Here's how the part is built. I have some questions about the finished solid (model axes, mm). A direction names the side the tool comes from. Coordinates: 2 decimals unless noted, no trailing zeros. Write each loop counter-clockwise with the first axis right and the second up, starting at its lowest first coordinate (ties: lowest second). Pieces come first, ordered by that corner, then holes. Notation, with made-up numbers: (44.25, 54) -> (103.25, 54) arc R25 ccw to (103.25, 70) -> close; hole circle Ø9 at (12.5, 56.5). An arc over 180 degrees is marked (long way). Use a Markdown table: item, result. Add a question column.
Item 1: Imagine slicing it at D-D, the plane z = 12. Write out the boundary of the cut face in (x, y), and give its area (3 significant figures).
Item 2: Imagine slicing it at C-C, the plane z = -13. Write out the boundary of the cut face in (x, y).
Item 3: If I drill on line 1 along X through (y, z) = (4.25, 1); line 2 along Y through (x, z) = (9, 8); line 3 along X through (y, z) = (7.5, -1.5), over which ranges is the centre line in solid material (lowest first)? Write a range as from..to.
Item 4: Imagine slicing it at A-A, the plane x = 0. Write out the boundary of the cut face in (y, z).
Item 5: Will these pins go through, and if not, where does the flat tip stop? pin 1 Ø2.5 at (y, z) = (7.5, 0.5) entering from -X; pin 2 Ø5 at (x, z) = (-12, 6.5) entering from +Y; pin 3 Ø6 at (y, z) = (7, -3) entering from +X.
Item 6: If we mould it in two halves opening along Z, with no side actions, what happens to faces 1 (the cylindrical face through (21.75, 6.45, -4.94)), 2 (the cylindrical face through (-20.66, 6.45, -1.75)), 3 (the flat face through (-30, 1, -9))? For each: pulls with the +Z half, pulls with the -Z half, needs draft (parallel to the pull), parting line crosses it, or undercut.
Item 7: Imagine slicing it at B-B, the plane y = 7.5. Write out the boundary of the cut face in (x, z), and give its area (3 significant figures).
Item 8: On a 3-axis mill with a long thin cutter (end or side, diameter ignored), from which of +Z, -Z, +X, -X, +Y, -Y can I reach the whole of each face in a straight line? I mean faces 4 (the flat face through (-27.7, 6, -5)), 5 (the flat face through (25.7, 6, -3)), 6 (the flat face through (27.7, 6, -5)), 7 (the cylindrical face through (0.609, 6.451, 27.693)), 8 (the flat face through (-15.214, 7, 0)). Say none if no direction works.
Autodesk Inventor part; units mm, degrees
ref_plane "YZ Plane" through (0, 0, 0) normal (1, 0, 0) x (0, 1, 0)
ref_plane "XZ Plane" through (0, 0, 0) normal (0, 1, 0) x (-1, 0, 0)
ref_plane "XY Plane" through (0, 0, 0) normal (0, 0, 1) x (1, 0, 0)
sketch "Sketch1" plane through (0, 0, 0) normal (0, 1, 0) x (-1, 0, 0)
  arc A0 (30, 0) -> (-30, 0) centre (0, 0) ccw
  line L0 (30, 0) -> (30, -18)
  line L1 (-30, 0) -> (-30, -18)
  arc A1 (30, -18) -> (-30, -18) centre (0, -34) ccw
  dimension "d0" = 60
  dimension "d1" = 34
  dimension "d4" = 18
extrude "Extrusion1" add sketch "Sketch1" along normal blind 3
sketch "Sketch2" plane through (0, 3, 0) normal (0, 1, 0) x (1, 0, 0)
  arc A0 (-30, 0) -> (30, 0) centre (0, 0) ccw
  arc A1 (-30, 18) -> (30, 18) centre (0, 34) ccw
  line L0 (-30, 18) -> (-30, 0)
  line L1 (30, 0) -> (30, 18)
  arc A2 (-27.7, 0) -> (27.7, 0) centre (0, 0) ccw
  line L2 (-27.7, 0) -> (-27.7, 10.5394)
  arc A3 (-27.7, 10.5394) -> (27.7, 10.5394) centre (0, 34) ccw
  line L3 (27.7, 10.5394) -> (27.7, 0)
  arc A4 (-25.7, 0) -> (25.7, 0) centre (0, 0) ccw
  line L4 (-25.7, 0) -> (-25.7, 5.6028)
  arc A5 (-25.7, 5.6028) -> (25.7, 5.6028) centre (0, 34) ccw
  line L5 (25.7, 5.6028) -> (25.7, 0)
  dimension "d5" = 2.3
  dimension "d6" = 2
extrude "Extrusion2" add sketch "Sketch2" along normal blind 7 contours L2 A3 L3 A2
sketch "Sketch3" plane through (0, 10, 0) normal (0, 1, 0) x (1, 0, 0)
  line L0 (-15.2137, -8.6006) -> (14.4909, -8.6006)
  line L1 (14.4909, -8.6006) -> (14.4909, 18.2853)
  line L2 (14.4909, 18.2853) -> (-15.2137, 18.2853)
  line L3 (-15.2137, 18.2853) -> (-15.2137, -8.6006)
  point P0 (0, 0)
extrude "Extrusion3" cut sketch "Sketch3" against normal blind 7
properties part number "Tapa general_3DPrint"
Ans:
| question | item | result |
|---|---|---|
| 1 | outline | (-27.5, 0) -> (27.5, 0) -> (27.5, 3) -> (24.97, 3) -> (24.97, 10) -> (22.73, 10) -> (22.73, 3) -> (-22.73, 3) -> (-22.73, 10) -> (-24.97, 10) -> (-24.97, 3) -> (-27.5, 3) -> close |
| 1 | area | 196 mm^2 |
| 2 | outline | (-30, 0) -> (-26.74, 0) -> (-26.74, 3) -> (-30, 3) -> close; (26.74, 0) -> (30, 0) -> (30, 3) -> (26.74, 3) -> close |
| 3 | line 1 | x = -27.68..-25.68, -15.55..-15.21, 14.49..15.55, 25.68..27.68 |
| 3 | line 2 | y = 0..3 |
| 3 | line 3 | x = -27.7..-25.7, -20.26..-16.17, 16.17..20.26, 25.7..27.7 |
| 4 | outline | (0, 0) -> (3, 0) -> (3, 25.7) -> (10, 25.7) -> (10, 27.7) -> (3, 27.7) -> (3, 30) -> (0, 30) -> close |
| 5 | pin 1 | stops at x = -27.7 |
| 5 | pin 2 | stops at y = 3 |
| 5 | pin 3 | stops at x = 27.7 |
| 6 | face 1 | pulls with the -Z half |
| 6 | face 2 | undercut |
| 6 | face 3 | needs draft |
| 7 | outline | (-27.7, -10.54) arc R36.3 cw to (-15.21, -1.04) -> (-15.21, 1.15) arc R38.3 ccw to (-25.7, -5.6) -> (-25.7, 0) arc R25.7 cw to (25.7, 0) -> (25.7, -5.6) arc R38.3 ccw to (14.49, 1.45) -> (14.49, -0.72) arc R36.3 cw to (27.7, -10.54) -> (27.7, 0) arc R27.7 ccw to (-27.7, 0) -> close |
| 7 | area | 258 mm^2 |
| 8 | face 4 | +Z, -Z, -X, +Y |
| 8 | face 5 | +Y |
| 8 | face 6 | +Z, -Z, +X, +Y |
| 8 | face 7 | +Z, +Y |
| 8 | face 8 | -Z, +Y |
